Read the model definition and answer for the solid it produces. Units are mm, in the model's axes. Face numbers are marked on the shaded views. A direction names the side the tool comes from. Round coordinates to 2 decimals unless told otherwise and drop trailing zeros. Loops run counter-clockwise (first coordinate to the right, second up) from the corner with the lowest first, then second, coordinate; pieces in that order, holes last. Notation, with made-up numbers: M -5,-16 L 46,-16 A12 cw 46,-4 Z; hole C 47,1.25 d9. An arc over 180 degrees is marked long. Answer as CSV lines item,"result".
```python
from build123d import *

# Parameters (mm, degrees)
SKETCH_1_W           = 30
SKETCH_1_H           = 13.5
EXTRUDE_1_DEPTH      = 20
SKETCH_2_W           = 10
SKETCH_2_H           = 20.163242361
CUT_EXTRUDE_2_DEPTH  = 29.41214529
SKETCH_3_R           = 3
CUT_EXTRUDE_3_DEPTH  = 37.827299657
SKETCH_6_W           = 30
SKETCH_6_H           = 13.5
EXTRUDE_5_DEPTH      = 10
SKETCH_7_R           = 3
CUT_EXTRUDE_1_DEPTH  = 29.41214529
SKETCH_9_W           = 6.52399098
SKETCH_9_H           = 33.458140235
CUT_EXTRUDE_6_DEPTH  = 29.41214529
SKETCH_14_W          = 84.903926308
SKETCH_14_H          = 44.963333207
CUT_EXTRUDE_10_DEPTH = 1
CHAMFER1_SIZE        = 10


with BuildPart() as part:
    # Эскиз1 → Вытянуть1 (new body)
    with BuildSketch(Plane.XY):
        with Locations((0, -0.75)):
            Rectangle(SKETCH_1_W, SKETCH_1_H)
    extrude(amount=EXTRUDE_1_DEPTH)

    # Эскиз2 → Вытянуть2 (cut, through all)
    with BuildSketch(Plane.XZ.offset(7.5)):
        with Locations((0, 18.081621181)):
            Rectangle(SKETCH_2_W, SKETCH_2_H)
    extrude(amount=-CUT_EXTRUDE_2_DEPTH, mode=Mode.SUBTRACT)

    # Эскиз3 → Вытянуть3 (cut, through all)
    with BuildSketch(Plane(origin=(15, 0, 0), x_dir=(0, 0, -1), z_dir=(1, 0, 0))):
        with Locations(Location((-14.861357689, 0, 0), (0, 0, 90))):
            Circle(SKETCH_3_R)
    extrude(amount=-CUT_EXTRUDE_3_DEPTH, mode=Mode.SUBTRACT)

    # Эскиз6 → Вытянуть5 (add)
    with BuildSketch(Plane(origin=(0, 0, 0), x_dir=(-1, 0, 0), z_dir=(0, 0, -1))):
        with Locations((0, -0.75)):
            Rectangle(SKETCH_6_W, SKETCH_6_H)
    extrude(amount=EXTRUDE_5_DEPTH)

    # Эскиз7 → Вырез-Вытянуть1 (cut, through all)
    with BuildSketch(Plane(origin=(0, 6, 0), x_dir=(1, 0, 0), z_dir=(0, 1, 0))):
        with Locations(Location((0.231400022, 0.869933179, 0), (0, 0, 270))):
            Circle(SKETCH_7_R)
    extrude(amount=-CUT_EXTRUDE_1_DEPTH, mode=Mode.SUBTRACT)

    # Эскиз9 → Вытянуть6 (cut, through all)
    with BuildSketch(Plane(origin=(0, 6, 0), x_dir=(1, 0, 0), z_dir=(0, 1, 0))):
        with Locations((16.26199549, -3.329208479)):
            Rectangle(SKETCH_9_W, SKETCH_9_H)
        with Locations((-16.26199549, -3.329208479)):
            Rectangle(SKETCH_9_W, SKETCH_9_H)
    extrude(amount=-CUT_EXTRUDE_6_DEPTH, mode=Mode.SUBTRACT)

    # Эскиз14 → Вытянуть10 (cut)
    with BuildSketch(Plane.XZ.offset(7.5)):
        with Locations((0.061866905, -0.327668242)):
            Rectangle(SKETCH_14_W, SKETCH_14_H)
    extrude(amount=-CUT_EXTRUDE_10_DEPTH, mode=Mode.SUBTRACT)

    # Chamfer1
    chamfer1_edges = [part.edges().sort_by_distance(p)[0] for p in [
        (-13, -0.25, -10),
        (13, -0.25, -10),
    ]]
    chamfer(chamfer1_edges, length=CHAMFER1_SIZE)


solid = part.part
```
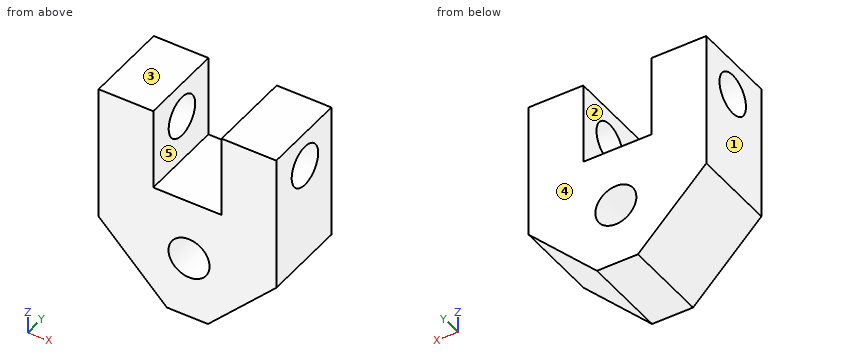
1) Determine the mould class of the marked faces 1, 2 and 3 for opening direction X: released by +X, released by -X, zero draft, split by the parting line, or undercut.
Evaluation:
face 1,"released by -X"
face 2,"undercut"
face 3,"zero draft"
2) Find section C-C, the plane y = -4.5. Give the vertices of the cut face in (x, z).
Evaluation:
outline,"M -13,0 L -3,-10 L 3,-10 L 13,0 L 13,20 L 5,20 L 5,8 L -5,8 L -5,20 L -13,20 Z; hole C 0.23,-0.87 d6"
3) A tool of negligible diameter and unlimited length cuts with its end or side. For the marked faces 4 and 5, from which of +Z, -Z, +X, -X, +Y, -Y can it reach the whole face along a straight path? Write none if from no direction.
Evaluation:
face 4,"+Z, -Z, +X, -X, +Y"
face 5,"+Z, +Y, -Y"
4) Find section D-D, the plane z = 12.25. Give the vertices of the cut face in (x, y).
Evaluation:
outline,"M -13,-6.5 L -5,-6.5 L -5,-1.48 L -13,-1.48 Z; M -13,1.48 L -5,1.48 L -5,6 L -13,6 Z; M 5,-6.5 L 13,-6.5 L 13,-1.48 L 5,-1.48 Z; M 5,1.48 L 13,1.48 L 13,6 L 5,6 Z"
5) Straight lines are drawn through the part: line 1 (X direction, y = -6, z = 15.5); line 2 (Y direction, x = -9.75, z = 14.75); line 3 (Z direction, x = -7, y = 0). For each, find the intervals that lie inside material, in ascending order.
Evaluation:
line 1,"x = -13 to -5, 5 to 13"
line 2,"y = -6.5 to -3, 3 to 6"
line 3,"z = -6 to 11.86, 17.86 to 20"
6) Find section A-A, the plane y = 0. Give the vertices of the cut face in (x, z).
Evaluation:
outline,"M -13,0 L -3,-10 L 3,-10 L 13,0 L 13,11.86 L 5,11.86 L 5,8 L -5,8 L -5,11.86 L -13,11.86 Z; M -13,17.86 L -5,17.86 L -5,20 L -13,20 Z; M 5,17.86 L 13,17.86 L 13,20 L 5,20 Z; hole C 0.23,-0.87 d6"
7) Find section B-B, the plane x = -1.5. Give the vertices of the cut face in (y, z), then the cut area to 3 significant figures.
Evaluation:
outline,"M -6.5,-10 L 6,-10 L 6,-3.32 L -6.5,-3.32 Z; M -6.5,1.58 L 6,1.58 L 6,8 L -6.5,8 Z"
area,"164 mm^2"
